from build123d import *

# Parameters (mm, degrees)
CYLINDER_R           = 1.3
CYLINDER_DEPTH       = 0.5
CYLINDER001_R        = 0.3
CYLINDER001_DEPTH    = 4
CYLINDER001001_R     = 0.3
CYLINDER001001_DEPTH = 4
BOX001001001_W       = 10.5
BOX001001001_H       = 3
BOX001001001_DEPTH   = 0.5
BOX001_W             = 7.5
BOX001_H             = 6
BOX001_DEPTH         = 0.5
BOX001001_W          = 10.5
BOX001001_H          = 3
BOX001001_DEPTH      = 0.5
BOX_W                = 8.5
BOX_H                = 4
BOX_DEPTH            = 8
FILLET_R             = 0.2


with BuildPart() as cylinder:
    # Cylinder → Cylinder (new body)
    with BuildSketch(Plane.XY):
        Circle(CYLINDER_R)
    extrude(amount=CYLINDER_DEPTH)


with BuildPart() as pin:
    # Cylinder001 → Cylinder001 (new body)
    with BuildSketch(Plane(origin=(-2.54, 0, -3.5), x_dir=(1, 0, 0), z_dir=(0, 0, 1))):
        Circle(CYLINDER001_R)
    extrude(amount=CYLINDER001_DEPTH)


with BuildPart() as pin001:
    # Cylinder001001 → Cylinder001001 (new body)
    with BuildSketch(Plane(origin=(2.54, 0, -3.5), x_dir=(1, 0, 0), z_dir=(0, 0, 1))):
        Circle(CYLINDER001001_R)
    extrude(amount=CYLINDER001001_DEPTH)


with BuildPart() as box001001001:
    # Box001001001 → Box001001001 (new body)
    with BuildSketch(Plane(origin=(-5.74, 1, 0), x_dir=(1, 0, 0), z_dir=(0, 0, 1))):
        with Locations((5.25, 1.5)):
            Rectangle(BOX001001001_W, BOX001001001_H)
    extrude(amount=BOX001001001_DEPTH)


with BuildPart() as box001:
    # Box001 → Box001 (new body)
    with BuildSketch(Plane(origin=(-3.74, -3, 0), x_dir=(1, 0, 0), z_dir=(0, 0, 1))):
        with Locations((3.75, 3)):
            Rectangle(BOX001_W, BOX001_H)
    extrude(amount=BOX001_DEPTH)


with BuildPart() as fusion:
    # Box001001 → Box001001 (new body)
    with BuildSketch(Plane(origin=(-5.74, -4, 0), x_dir=(1, 0, 0), z_dir=(0, 0, 1))):
        with Locations((5.25, 1.5)):
            Rectangle(BOX001001_W, BOX001001_H)
    extrude(amount=BOX001001_DEPTH)

    # Fusion: union Box001001001, Box001
    add(box001001001.part)
    add(box001.part)


with BuildPart() as obj1:
    # Box → Box (new body)
    with BuildSketch(Plane(origin=(-4.24, -2, 0), x_dir=(1, 0, 0), z_dir=(0, 0, 1))):
        with Locations((4.25, 2)):
            Rectangle(BOX_W, BOX_H)
    extrude(amount=BOX_DEPTH)

    # Cut: cut Fusion
    add(fusion.part, mode=Mode.SUBTRACT)

    # Fillet
    fillet_edges = [obj1.edges().sort_by_distance(p)[0] for p in [
        (-4.24, 0, 8),
        (0.01, 2, 8),
        (4.26, 0, 8),
        (0.01, -2, 8),
        (-4.24, -2, 4.25),
        (-4.24, 2, 4.25),
        (4.26, 2, 4.25),
        (4.26, -2, 4.25),
    ]]
    fillet(fillet_edges, radius=FILLET_R)

    # Fusion001: union Cylinder, PIN, PIN001
    add(cylinder.part)
    add(pin.part)
    add(pin001.part)


solid = obj1.part
CAD build for the part. Positions are in the model's coordinates, mm. A direction names the side the tool comes from. Coordinates: 2 decimals unless noted, no trailing zeros. Write each loop counter-clockwise with the first axis right and the second up, starting at its lowest first coordinate (ties: lowest second). Pieces come first, ordered by that corner, then holes. Notation, with made-up numbers: M 21,15 L 49,15 A30 ccw 49,42 Z; hole C 13,83.25 d5. An arc over 180 degrees is marked long. Answer as a JSON object with one key per item and string values. Group by question number.
1) Saw through at C-C (y = 0). Write the cut outline in (x, z).
2) Tool access for faces 4 (the face through (0, 0, 0)), 5 (the face through (-0.17, 1.29, 0.25)), 6 (the face through (0, 2, 4)): list every direction of +Z, -Z, +X, -X, +Y, -Y with a clear straight run to the whole face (end or side of a thin tool).
3) Saw through at A-A (z = 0.25). Write the cut outline in (x, y), plus the area to 3 significant figures.
4) Wall check: line 1 (Z direction, x = -1.5, y = -0.35); line 2 (Z direction, x = 1, y = -0.3); line 3 (X direction, y = 0.05, z = -2.75). Give the ranges that are in metal, low to high. Write a range as from..to.
5) Saw through at B-B (x = -2.54). Write the cut outline in (y, z), plus the area to 3 significant figures.
6) Pin check, flat tips, straight feed: pin 1 Ø2 at (x, y) = (0, -0.5) entering from -Z; pin 2 Ø0.6 at (x, z) = (4, 0) entering from +Y. Stop position of each tip, or through.
7) Saw through at D-D (x = 0). Write the cut outline in (y, z).
8) Mould opens along X. For faces 1 (the face through (-4.24, 0, 4)), 2 (the face through (0, -2, 4)), 3 (the face through (0.9, 1.4, 0.5)) say: +X half, -X half, draft (parallel to the pull), parting line (faces both ways), or undercut.
Values follow:
{
 "1": {"outline": "M -4.24,0 L -3.74,0 L -3.74,0.5 L -2.84,0.5 L -2.84,-3.5 L -2.24,-3.5 L -2.24,0.5 L -1.3,0.5 L -1.3,0 L 1.3,0 L 1.3,0.5 L 2.24,0.5 L 2.24,-3.5 L 2.84,-3.5 L 2.84,0.5 L 3.76,0.5 L 3.76,0 L 4.26,0 L 4.26,7.8 A0.2 ccw 4.06,8 L -4.04,8 A0.2 ccw -4.24,7.8 Z"},
 "2": {"face 4": "-Z, +Y, -Y", "face 5": "-Z", "face 6": "+Z, -Z, +X, -X, +Y"},
 "3": {"outline": "M -4.24,-1 L -3.74,-1 L -3.74,1 L -4.24,1 Z; C -2.54,0 d0.6; C 0,0 d2.6; C 2.54,0 d0.6; M 3.76,-1 L 4.26,-1 L 4.26,1 L 3.76,1 Z", "area": "7.87 mm2"},
 "4": {"line 1": "z = 0.5..8", "line 2": "z = 0..8", "line 3": "x = -2.84..-2.24, 2.24..2.84"},
 "5": {"outline": "M -2,0.5 L -0.3,0.5 L -0.3,-3.5 L 0.3,-3.5 L 0.3,0.5 L 2,0.5 L 2,7.8 A0.2 ccw 1.8,8 L -1.8,8 A0.2 ccw -2,7.8 Z", "area": "32.4 mm2"},
 "6": {"pin 1": "stops at z = 0", "pin 2": "stops at y = 1"},
 "7": {"outline": "M -2,0.5 L -1.3,0.5 L -1.3,0 L 1.3,0 L 1.3,0.5 L 2,0.5 L 2,7.8 A0.2 ccw 1.8,8 L -1.8,8 A0.2 ccw -2,7.8 Z"},
 "8": {"face 1": "-X half", "face 2": "draft", "face 3": "undercut"}
}
